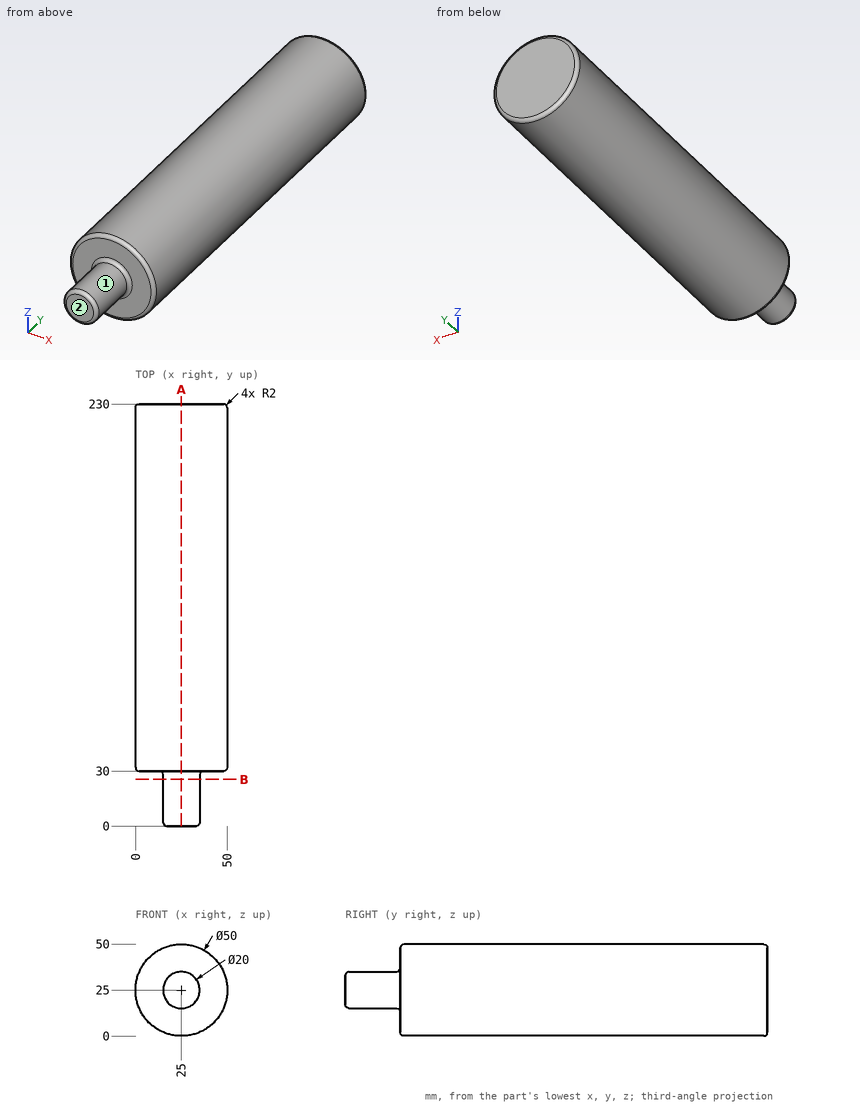
Source: three-view drawing plus pictorial views. Frame: mm from the lowest corner of the part. A direction names the side the tool comes from. Round coordinates to 2 decimals unless told otherwise and drop trailing zeros. Write each loop counter-clockwise with the first axis right and the second up, starting at its lowest first coordinate (ties: lowest second). Pieces come first, ordered by that corner, then holes. Notation, with made-up numbers: M 85.5,68.5 L 105.5,68.5 A22 ccw 105.5,87.5 Z; hole C 39,64 d1. An arc over 180 degrees is marked long. Write each question's results on one line, items separated by ' | '.
Q1. Section query A-A (x = 25). Return loops of the section in (y, z).
Results:
outline: M 0,17 A2 ccw 2,15 L 28,15 A2 cw 30,13 L 30,2 A2 ccw 32,0 L 228,0 A2 ccw 230,2 L 230,48 A2 ccw 228,50 L 32,50 A2 ccw 30,48 L 30,37 A2 cw 28,35 L 2,35 A2 ccw 0,33 Z
Q2. Access query for the marked faces 1 and 2. Directions: +Z, -Z, +X, -X, +Y, -Y. A direction counts if a zero-diameter tool reaches every point of the face in a straight line with its end or side. Return the directions, or none.
Results:
face 1: -Y | face 2: +Z, -Z, +X, -X, -Y
Q3. Section query B-B (y = 25.5). Return loops of the section in (x, z).
Results:
outline: C 25,25 d20
Q4. Line query: line 1 along Y through (x, z) = (13, 6.5); line 2 along Z through (x, y) = (25.5, 206) (3 decimals); line 3 along X through (y, z) = (48, 23.5). Output: solid intervals per line, ascending.
Results:
line 1: y = 30 to 230 | line 2: z = 0.005 to 49.995 | line 3: x = 0.05 to 49.95
Q5. Pin query (flat end, axial travel): P1, Ø5, axis at x = 9.5, y = 92, coming from the -Z side; P2, Ø10, axis at y = 109, z = 6.5, coming from the -X side; P3, Ø8, axis at x = 32, z = 39.5, coming from the -Y side. Return the tip coordinate at first contact, or that it passes through.
Results:
P1: stops at z = 3.65 | P2: stops at x = 3.96 | P3: stops at y = 30
